Design review of the part built by this model. Coordinates are the model's own, in mm. Face numbers are marked on the shaded views. A direction names the side the tool comes from. Coordinates: 2 decimals unless noted, no trailing zeros. Order: outer loops, then holes, each group sorted by start corner. A loop starts at its lowest first (then second) coordinate and runs counter-clockwise, first axis right, second up. Notation, with made-up numbers: (23, -26.5) -> (32, -26.5) arc R22 ccw to (32, 6.5) -> close; hole circle Ø8 at (-19.5, 16.25). An arc over 180 degrees is marked (long way). Use a Markdown table: item, result. Add a question column.
Q1. Insertion check: pin 1 (3 mm diameter, centred on y = -1.5, z = 6, fed in from +X); pin 2 (5 mm diameter, centred on x = -3, y = 0, fed in from -Z); pin 3 (8 mm diameter, centred on y = -3, z = -10.5, fed in from +X). Each pin has a flat end and moves straight along its axis. Give the tip position at first contact, or say it passes through.
Q2. Machinability: for the marked faces 4 and 5, which of the approach directions +Z, -Z, +X, -X, +Y, -Y give a long, thin tool a straight path to every point of the face, cutting with its end or side? Answer none if there is none.
Q3. Add section B-B (z = -1.5). State the section outline as (x, y) points, then the cut area to 3 significant figures.
Q4. Add section A-A (x = 0). State the section outline as (y, z) points.
Q5. Wall thickness on probe 1 along X at (y, z) = (-5.2, 0); probe 2 along X at (y, z) = (4.6, 0); probe 3 along Y at (x, z) = (10.5, -14.5): over which ranges is each line inside the solid? List them lowest first.
Q6. The part is to be moulded in two halves that separate along Z. For the marked faces 1, 2 and 3, say which applies: pulls with the +Z half, pulls with the -Z half, needs draft (parallel to the pull), parting line crosses it, or undercut.
Q7. Add section D-D (y = 6.25). Count the separate pieces of the cut face and the enclosed holes in it, then the cut area to 3 significant figures.
Q8. Add section C-C (z = 19). State the section outline as (x, y) points.
from build123d import *

# Parameters (mm, degrees)
IZIM1_R                     = 47.5
Y_KSEKLIK_EKSTR_ZYON1_DEPTH = 7.75
IZIM2_OUTSIDE_W             = 124.048
IZIM2_OUTSIDE_H             = 124.048
IZIM2_OUTSIDE_R             = 32.5
KES_EKSTR_ZYON1_DEPTH       = 8
KES_EKSTR_ZYON2_DEPTH       = 10.5
IZIM4_R                     = 30
KES_EKSTR_ZYON3_DEPTH       = 6
IZIM5_R                     = 1.5
KES_EKSTR_ZYON4_DEPTH       = 69.940191471
DAIRESEL_KAPLAMA1_COUNT     = 8
IZIM6_R                     = 7.5
KES_EKSTR_ZYON5_DEPTH       = 69.940191471


with BuildPart() as part:
    # Çizim1 → Yükseklik-Ekstrüzyon1 (new, symmetric)
    with BuildSketch(Plane(origin=(0, 0, 0), x_dir=(1, 0, 0), z_dir=(0, 1, 0))):
        with Locations(Location((0, 0, 0), (0, 0, 270))):
            Circle(IZIM1_R)
    extrude(amount=Y_KSEKLIK_EKSTR_ZYON1_DEPTH, both=True)

    # Çizim2 outside → Kes-Ekstrüzyon1 (cut)
    with BuildSketch(Plane.XZ.offset(7.75)):
        Rectangle(IZIM2_OUTSIDE_W, IZIM2_OUTSIDE_H)
        with Locations(Location((0, 0, 0), (0, 0, 270))):
            Circle(IZIM2_OUTSIDE_R, mode=Mode.SUBTRACT)
    extrude(amount=-KES_EKSTR_ZYON1_DEPTH, mode=Mode.SUBTRACT)

    # Çizim3 → Kes-Ekstrüzyon2 (cut)
    with BuildSketch(Plane.XZ.offset(7.75)):
        Polygon((15.25, 0), (7.625, 13.206887408), (-7.625, 13.206887408), (-15.25, 0), (-7.625, -13.206887408), (7.625, -13.206887408), align=None)
    extrude(amount=-KES_EKSTR_ZYON2_DEPTH, mode=Mode.SUBTRACT)

    # Çizim4 → Kes-Ekstrüzyon3 (cut)
    with BuildSketch(Plane.XZ.offset(7.75)):
        with Locations(Location((0, 0, 0), (0, 0, 270))):
            Circle(IZIM4_R)
    extrude(amount=-KES_EKSTR_ZYON3_DEPTH, mode=Mode.SUBTRACT)

    # Çizim5 → Kes-Ekstrüzyon4 (cut, through all)
    with BuildSketch(Plane(origin=(0, 7.75, 0), x_dir=(1, 0, 0), z_dir=(0, 1, 0))):
        with Locations(Location((-16.264045876, 39.264880132, 0), (0, 0, 270))):
            Circle(IZIM5_R)
    kes_ekstr_zyon4 = extrude(amount=-KES_EKSTR_ZYON4_DEPTH, mode=Mode.SUBTRACT)

    # Dairesel Kaplama1: Kes-Ekstrüzyon4 ×8 about axis
    dairesel_kaplama1_axis = Axis((0, 0, 0), (0, 1, 0))
    for i in range(1, DAIRESEL_KAPLAMA1_COUNT):
        add(kes_ekstr_zyon4.rotate(dairesel_kaplama1_axis, i * 360 / DAIRESEL_KAPLAMA1_COUNT), mode=Mode.SUBTRACT)

    # Çizim6 → Kes-Ekstrüzyon5 (cut, through all)
    with BuildSketch(Plane(origin=(0, 7.75, 0), x_dir=(1, 0, 0), z_dir=(0, 1, 0))):
        with Locations(Location((0, 0, 0), (0, 0, 270))):
            Circle(IZIM6_R)
    extrude(amount=-KES_EKSTR_ZYON5_DEPTH, mode=Mode.SUBTRACT)


solid = part.part
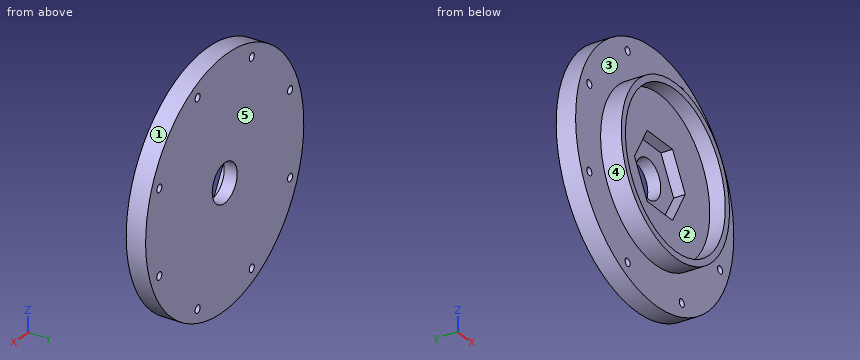
Established:
| question | item | result |
|---|---|---|
| 1 | pin 1 | x = 32.19 |
| 1 | pin 2 | z = -47.5 |
| 1 | pin 3 | x = 46.79 |
| 2 | face 4 | -Y |
| 2 | face 5 | +Z, -Z, +X, -X, +Y |
| 3 | outline | (-47.48, 0.25) -> (-32.47, 0.25) -> (-32.47, -7.75) -> (-29.96, -7.75) -> (-29.96, -1.75) -> (-14.38, -1.75) -> (-14.38, 2.75) -> (-7.35, 2.75) -> (-7.35, 7.75) -> (-47.48, 7.75) -> close; (7.35, 2.75) -> (14.38, 2.75) -> (14.38, -1.75) -> (29.96, -1.75) -> (29.96, -7.75) -> (32.47, -7.75) -> (32.47, 0.25) -> (47.48, 0.25) -> (47.48, 7.75) -> (7.35, 7.75) -> close |
| 3 | area | 669 mm^2 |
| 4 | outline | (-7.75, -32.5) -> (0.25, -32.5) -> (0.25, -47.5) -> (7.75, -47.5) -> (7.75, -7.5) -> (2.75, -7.5) -> (2.75, -13.21) -> (-1.75, -13.21) -> (-1.75, -30) -> (-7.75, -30) -> close; (-7.75, 30) -> (-1.75, 30) -> (-1.75, 13.21) -> (2.75, 13.21) -> (2.75, 7.5) -> (7.75, 7.5) -> (7.75, 47.5) -> (0.25, 47.5) -> (0.25, 32.5) -> (-7.75, 32.5) -> close |
| 5 | probe 1 | -32.5 to -30, 30 to 32.5 |
| 5 | probe 2 | -47.5 to -7.5, 7.5 to 47.5 |
| 5 | probe 3 | -1.75 to 7.75 |
| 6 | face 1 | parting line crosses it |
| 6 | face 2 | undercut |
| 6 | face 3 | needs draft |
| 7 | separate pieces | 1 |
| 7 | enclosed holes | 9 |
| 7 | area | 6,850 mm^2 |
| 8 | outline | (-43.53, 0.25) -> (-26.37, 0.25) -> (-26.37, -7.75) -> (-23.22, -7.75) -> (-23.22, -1.75) -> (23.22, -1.75) -> (23.22, -7.75) -> (26.37, -7.75) -> (26.37, 0.25) -> (43.53, 0.25) -> (43.53, 7.75) -> (-43.53, 7.75) -> close |
